Here's the drawing with two shaded views (mm, measured from the low corner). I have some questions. Give positions to 0.01 mm unless a question says otherwise; leave off trailing zeros. Loops run counter-clockwise (first coordinate to the right, second up) from the corner with the lowest first, then second, coordinate; pieces in that order, holes last. Notation, with made-up numbers: M -36,34 L -19,34 A26 cw -19,72 Z; hole C 53,44 d7. An arc over 180 degrees is marked long. Use a Markdown table: item, result. Add a question column.
1) Suppose I cut it at A-A on z = 22.5. List the corners of the cut face in (x, y) for me (1 decimal).
2) Suppose I cut it at D-D on z = 32. List the corners of the cut face in (x, y) for me (1 decimal).
3) If I drill on line 1 along Z through (x, y) = (22, 0.8) (1 decimal); line 2 along X through (y, z) = (0.9, 21) (1 decimal); line 3 along X through (y, z) = (0.5, 12), over which ranges is the centre line in solid material (lowest first)? Write a range as [from, to].
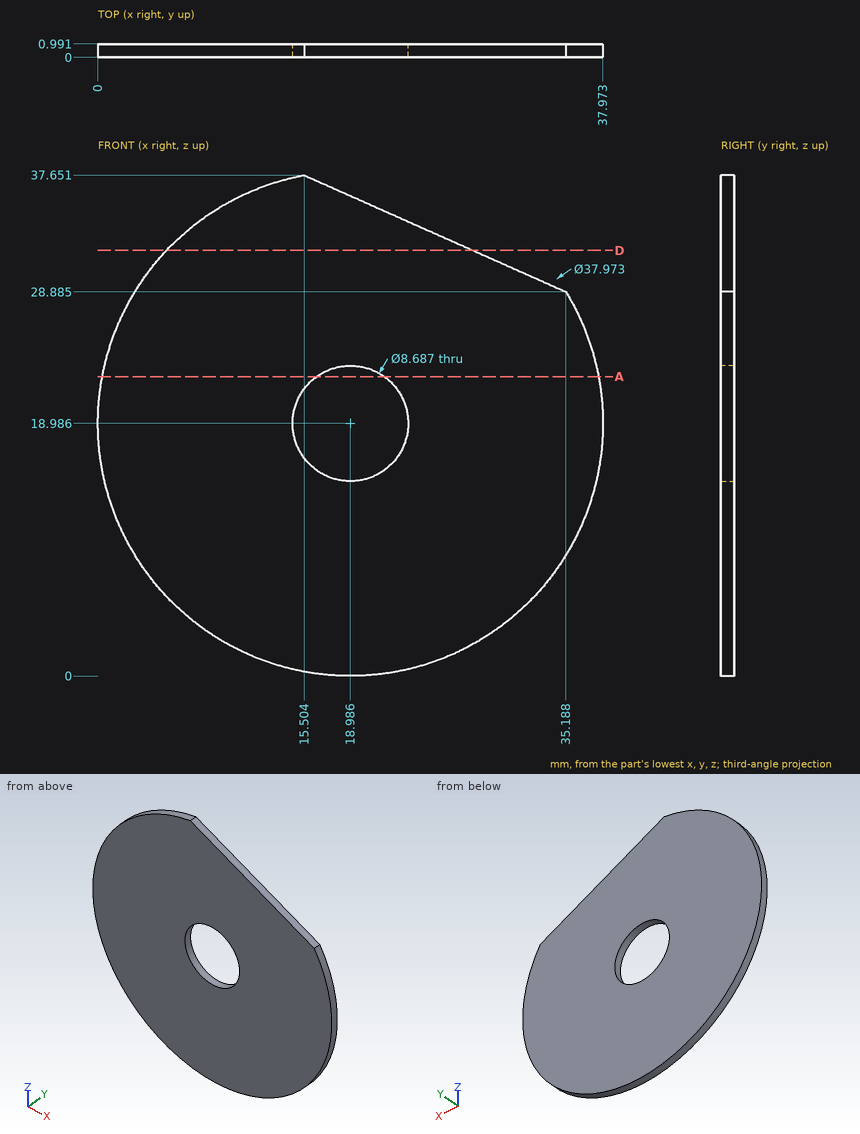
Answer block:
| question | item | result |
|---|---|---|
| 1 | outline | M 0.3,0 L 16.4,0 L 16.4,1 L 0.3,1 Z; M 21.5,0 L 37.6,0 L 37.6,1 L 21.5,1 Z |
| 2 | outline | M 5.2,0 L 28.2,0 L 28.2,1 L 5.2,1 Z |
| 3 | line 1 | z = [0.2, 15.9], [22.1, 34.8] |
| 3 | line 2 | x = [0.1, 15.1], [22.8, 37.9] |
| 3 | line 3 | x = [1.33, 36.64] |
